The listing builds one solid part. Answer for the finished solid, in the listing's coordinates (mm). Round coordinates to 2 decimals unless told otherwise and drop trailing zeros. Order: outer loops, then holes, each group sorted by start corner. A loop starts at its lowest first (then second) coordinate and runs counter-clockwise, first axis right, second up. Notation, with made-up numbers: (76.5, 79.25) -> (117.5, 79.25) arc R24 ccw to (117.5, 92.25) -> close; hole circle Ø4 at (45, 24). An arc over 180 degrees is marked (long way). Return JSON: item names as keys, results as strings. Group by question number.
(1) The part is cut by section B-B (z = 34.5). Determine the outline of the cut face in (x, y), plus the area to 3 significant figures.
(2) Consider line 1 (Z direction, x = -64.5, y = 88); line 2 (Z direction, x = -21.5, y = 25.5). Determine where each line is inside the solid, lowest interval first. Write a range as [from, to].
(3) The part is cut by section D-D (y = 70). Determine the outline of the cut face in (x, z), plus the area to 3 significant figures.
(4) Each of these flat-tipped pins is pushed along its axis until it touches: pin 1 (8 mm diameter, centred on y = 65.5, z = -73.5, fed in from +X); pin 2 (0.5 mm diameter, centred on x = 3, z = -19.5, fed in from +Y); pin 3 (9 mm diameter, centred on y = 37, z = 23, fed in from -X). Where does it stop, or does it pass through?
(5) The part is cut by section C-C (x = -39). Determine the outline of the cut face in (y, z), plus the area to 3 significant figures.
(6) The part is cut by section A-A (y = 168.5). Determine the outline of the cut face in (x, z), plus the area to 3 significant figures.
from build123d import *

# Parameters (mm, degrees)
SALIENTE_EXTRUIR1_DEPTH = 2.5
SALIENTE_EXTRUIR2_DEPTH = 4
MATRIZC2_COUNT          = 4
CHAFL_N1_SIZE           = 2


with BuildPart() as part:
    # Croquis2 → Revoluci_n1 (revolve)
    with BuildSketch(Plane.XY, mode=Mode.PRIVATE) as revoluci_n1_sk:
        with BuildLine():
            Line((0, 0), (0, 615))
            ThreePointArc((0, 615), (13.099961221, 558.161950621), (17.5, 500))
            Line((17.5, 500), (17.5, 0))
            Line((17.5, 0), (0, 0))
        make_face()
    revolve(revoluci_n1_sk.sketch.rotate(Axis((0, 0, 0), (0, 1, 0)), 90), axis=Axis((0, 0, 0), (0, 1, 0)))

    # Croquis3 → Saliente-Extruir1 (add, symmetric)
    with BuildSketch(Plane.XY):
        Polygon((0, 10), (-97.579043475, 30.741065972), (-97.579043475, 50.741065972), (0, 260), align=None)
    saliente_extruir1 = extrude(amount=SALIENTE_EXTRUIR1_DEPTH, both=True)

    # Croquis4 → Saliente-Extruir2 (add, symmetric)
    with BuildSketch(Plane.XY):
        Polygon((-25, 15.313914042), (-25, 60.313914042), (0, 60.313914042), (0, 10), align=None)
    saliente_extruir2 = extrude(amount=SALIENTE_EXTRUIR2_DEPTH, both=True)

    # MatrizC2: Saliente-Extruir1, Saliente-Extruir2 ×4 about axis
    matrizc2_axis = Axis((0, 0, 0), (0, 1, 0))
    add([saliente_extruir1.rotate(matrizc2_axis, i * 360 / MATRIZC2_COUNT) for i in range(1, MATRIZC2_COUNT)])
    add([saliente_extruir2.rotate(matrizc2_axis, i * 360 / MATRIZC2_COUNT) for i in range(1, MATRIZC2_COUNT)])

    # Chafl_n1
    chafl_n1_edges = [part.edges().sort_by_distance(p)[0] for p in [
        (0, 0, 17.5),
    ]]
    chamfer(chafl_n1_edges, length=CHAFL_N1_SIZE)


solid = part.part
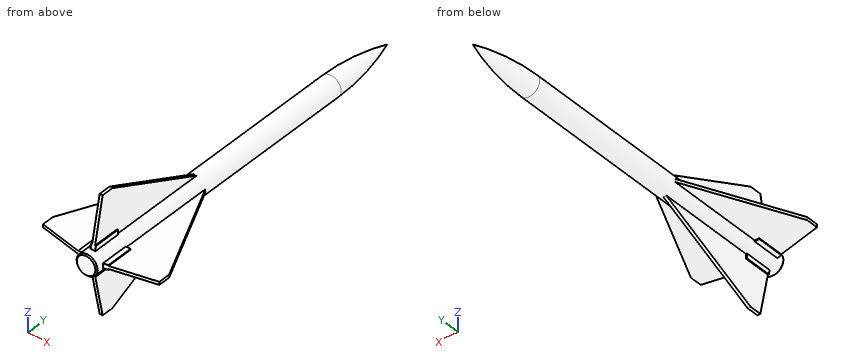
Answer below:
{
 "1": {"outline": "(-2.5, 17.33) -> (2.5, 17.33) -> (2.5, 186.01) -> (-2.5, 186.01) -> close", "area": "843 mm²"},
 "2": {"line 1": "z = [-2.5, 2.5]", "line 2": "z = [-4, 4]"},
 "3": {"outline": "(-88.6, -2.5) -> (-17.32, -2.5) arc R17.5 ccw to (-2.5, -17.32) -> (-2.5, -88.6) -> (2.5, -88.6) -> (2.5, -17.32) arc R17.5 ccw to (17.32, -2.5) -> (88.6, -2.5) -> (88.6, 2.5) -> (17.32, 2.5) arc R17.5 ccw to (2.5, 17.32) -> (2.5, 88.6) -> (-2.5, 88.6) -> (-2.5, 17.32) arc R17.5 ccw to (-17.32, 2.5) -> (-88.6, 2.5) -> close", "area": "2,390 mm²"},
 "4": {"pin 1": "stops at x = 2.5", "pin 2": "stops at y = 60.31", "pin 3": "stops at x = -4"},
 "5": {"outline": "(18.29, -2.5) -> (176.36, -2.5) -> (176.36, 2.5) -> (18.29, 2.5) -> close", "area": "790 mm²"},
 "6": {"outline": "(-42.67, -2.5) -> (-17.32, -2.5) arc R17.5 ccw to (-2.5, -17.32) -> (-2.5, -42.67) -> (2.5, -42.67) -> (2.5, -17.32) arc R17.5 ccw to (17.32, -2.5) -> (42.67, -2.5) -> (42.67, 2.5) -> (17.32, 2.5) arc R17.5 ccw to (2.5, 17.32) -> (2.5, 42.67) -> (-2.5, 42.67) -> (-2.5, 17.32) arc R17.5 ccw to (-17.32, 2.5) -> (-42.67, 2.5) -> close", "area": "1,470 mm²"}
}
